Autodesk Inventor part; units mm, degrees
ref_plane "YZ Plane" through (0, 0, 0) normal (1, 0, 0) x (0, 1, 0)
ref_plane "XZ Plane" through (0, 0, 0) normal (0, 1, 0) x (-1, 0, 0)
ref_plane "XY Plane" through (0, 0, 0) normal (0, 0, 1) x (1, 0, 0)
sketch "Sketch1" plane through (0, 0, 0) normal (0, 1, 0) x (-1, 0, 0)
  line L0 (-17.15, 21.15) -> (17.15, 21.15)
  line L1 (21.15, 17.15) -> (21.15, -17.15)
  line L2 (17.15, -21.15) -> (-17.15, -21.15)
  line L3 (-21.15, -17.15) -> (-21.15, 17.15)
  line L4 (-21.15, 21.15) -> (21.15, -21.15) construction
  line L5 (21.15, 21.15) -> (-21.15, -21.15) construction
  line L6 (-15.5, 15.5) -> (15.5, 15.5)
  line L7 (15.5, 15.5) -> (15.5, -15.5)
  line L8 (15.5, -15.5) -> (-15.5, -15.5)
  line L9 (-15.5, -15.5) -> (-15.5, 15.5)
  line L10 (-15.5, 15.5) -> (15.5, -15.5) construction
  line L11 (15.5, 15.5) -> (-15.5, -15.5) construction
  circle A0 centre (15.5, 15.5) radius 1.5
  circle A1 centre (-15.5, 15.5) radius 1.5
  circle A2 centre (15.5, -15.5) radius 1.5
  circle A3 centre (-15.5, -15.5) radius 1.5
  line L12 (21.15, 17.15) -> (17.15, 21.15)
  line L13 (-21.15, 17.15) -> (-17.15, 21.15)
  line L14 (-17.15, -21.15) -> (-21.15, -17.15)
  line L15 (17.15, -21.15) -> (21.15, -17.15)
  point P0 (0, 0)
  dimension "d0" = 42.3
  dimension "d1" = 42.3
  dimension "d2" = 31
  dimension "d3" = 31
  dimension "d4" = 3
  dimension "d7" = 31
  dimension "d10" = 31
  dimension "d13" = 4
  dimension "d14" = 4
  dimension "d15" = 4
  dimension "d16" = 4
  dimension "d17" = 4
  dimension "d18" = 4
  dimension "d19" = 4
  dimension "d20" = 4
extrude "Extrusion1" add sketch "Sketch1" along normal blind 34 contours L0 L12 L1 L15 L2 L14 L3 L13 | L6 A0 L7 A2 L8 A3 L9 A1
sketch "Sketch2" plane through (0, 34, 0) normal (0, 1, 0) x (1, 0, 0)
  circle A0 centre (0, 0) radius 11
  dimension "d23" = 22
extrude "Extrusion2" add sketch "Sketch2" along normal blind 2
sketch "Sketch3" plane through (0, 36, 0) normal (0, 1, 0) x (1, 0, 0)
  circle A0 centre (0, 0) radius 2.5
  dimension "d26" = 5
extrude "Extrusion3" add sketch "Sketch3" along normal blind 24
chamfer "Chamfer1" distance 0.5 angle 45 1 edges at (-2.5, 60, 0)
sketch "Sketch4" plane through (-17.15, 0, 21.15) normal (0, 0, 1) x (1, 0, 0)
  line L0 (13.15, 0) -> (21.15, 0)
  line L1 (0, 0) -> (34.3, 0)
  line L2 (21.15, 0) -> (13.15, 0)
  line L3 (13.15, 0) -> (13.15, 6)
  line L4 (13.15, 6) -> (21.15, 6)
  line L5 (21.15, 6) -> (21.15, 0)
  point P0 (17.15, 0)
  dimension "d32" = 8
  dimension "d33" = 8
  dimension "d34" = 6
extrude "Extrusion4" add sketch "Sketch4" along normal blind 2
equation "\"d14\" = d13"
equation "\"d15\" = d13"
equation "\"d16\" = d15"
equation "\"d17\" = d13"
equation "\"d18\" = d17"
equation "\"d19\" = d13"
equation "\"d20\" = d19"
properties part number "Stepper_motor"
CAD build for the part. Positions are in the model's coordinates, mm. A direction names the side the tool comes from. Coordinates: 2 decimals unless noted, no trailing zeros. Order: outer loops, then holes, each group sorted by start corner. A loop starts at its lowest first (then second) coordinate and runs counter-clockwise, first axis right, second up. Notation, with made-up numbers: (3, 68) - (33, 68) arc R35 ccw to (33, 107) - close; hole circle Ø3 at (4, 87.25). An arc over 180 degrees is marked (long way). Answer in a Markdown table with one row per item.
1. Pull direction Z, two halves, no side cores. Call faces 1 (the face through (17, 16.76, 15.43)), 2 (the face through (0, 6, 22)), 3 (the face through (-2.38, 34.99, -10.74)): +Z half, -Z half, draft (parallel to the pull), parting line (faces both ways), or undercut.
Answer:
| item | result |
|---|---|
| face 1 | undercut |
| face 2 | draft |
| face 3 | parting line |
2. 3-axis set-ups, long thin cutter, end or side, ignore diameter. For faces 4 (the face through (4, 3, 22)), 5 (the face through (-0.54, 47.59, -2.44)), 6 (the face through (-4, 3, 22)): which of +Z, -Z, +X, -X, +Y, -Y reach the whole face in a straight line?
Answer:
| item | result |
|---|---|
| face 4 | +Z, +X, +Y, -Y |
| face 5 | +Y |
| face 6 | +Z, -X, +Y, -Y |
3. Slice it at B-B, the plane x = 15.5. List the corners of the cut face in (y, z).
Answer:
| item | result |
|---|---|
| outline | (0, -21.15) - (34, -21.15) - (34, -17) - (0, -17) - close; (0, -14) - (34, -14) - (34, 14) - (0, 14) - close; (0, 17) - (34, 17) - (34, 21.15) - (0, 21.15) - close |
4. Slice it at A-A, the plane z = -15.5. List the corners of the cut face in (x, y).
Answer:
| item | result |
|---|---|
| outline | (-21.15, 0) - (-17, 0) - (-17, 34) - (-21.15, 34) - close; (-14, 0) - (14, 0) - (14, 34) - (-14, 34) - close; (17, 0) - (21.15, 0) - (21.15, 34) - (17, 34) - close |
5. Drill centre lines: L1, parallel to Z at x = 15.5, y = 8.5; L2, parallel to Z at x = -15, y = 9. Where is each one in solid material? Low to high. Write a range as from..to.
Answer:
| item | result |
|---|---|
| L1 | -21.15..-17, -14..14, 17..21.15 |
| L2 | -21.15..-16.91, -14.09..14.09, 16.91..21.15 |
6. Slice it at D-D, the plane z = 0. List the corners of the cut face in (x, y), then the cut area to 3 significant figures.
Answer:
| item | result |
|---|---|
| outline | (-21.15, 0) - (21.15, 0) - (21.15, 34) - (11, 34) - (11, 36) - (2.5, 36) - (2.5, 59.5) - (2, 60) - (-2, 60) - (-2.5, 59.5) - (-2.5, 36) - (-11, 36) - (-11, 34) - (-21.15, 34) - close |
| area | 1,600 mm² |
7. Slice it at C-C, the plane y = 27. List the corners of the cut face in (x, z), then the cut area to 3 significant figures.
Answer:
| item | result |
|---|---|
| outline | (-21.15, -17.15) - (-17.15, -21.15) - (17.15, -21.15) - (21.15, -17.15) - (21.15, 17.15) - (17.15, 21.15) - (-17.15, 21.15) - (-21.15, 17.15) - close; hole circle Ø3 at (-15.5, -15.5); hole circle Ø3 at (-15.5, 15.5); hole circle Ø3 at (15.5, -15.5); hole circle Ø3 at (15.5, 15.5) |
| area | 1,730 mm² |
8. Flat gauge pins, fed straight in: P1, Ø5, axis at x = 13.5, y = 35.5, coming from the +Z side; P2, Ø12, axis at x = -2, z = 9.5, coming from the +Y side; P3, Ø1, axis at y = 4, z = 22, coming from the +X side. Where does each tip first touch, or does it go through?
Answer:
| item | result |
|---|---|
| P1 | z = 21.15 |
| P2 | y = 36 |
| P3 | x = 4 |
